Check sheet for the modelled part. Datum: model origin and axes. Units: mm. A direction names the side the tool comes from. Round coordinates to 2 decimals unless told otherwise and drop trailing zeros. Order: outer loops, then holes, each group sorted by start corner. A loop starts at its lowest first (then second) coordinate and runs counter-clockwise, first axis right, second up.
(1) Mould release check, pull along Y, two halves, no side actions. Record for faces 4 (the cylindrical face through (46.536, 9.274, 7.675)), 5 (the flat face through (34, 0, -1)), 6 (the cylindrical face through (24.5, 5.6, -5.6)): released by +Y, released by -Y, zero draft, split by the parting line, or undercut.
(2) Tool access check on faces 1 (the flat face through (10, 5.4, -8.5)), 2 (the flat face through (44, 2, 4)), 3 (the flat face through (31, 5, -11)). Record the directions out of +Z, -Z, +X, -X, +Y, -Y that give a thin tool (end or side, any length) a straight path to the whole face; none if there is none.
(3) Thickness scan on probe 1 along Y at (x, z) = (51, 5.75); probe 2 along X at (y, z) = (2.35, 8); probe 3 along Y at (x, z) = (40, -6). Record the ranges inside material, lowest first.
(4) Sectioned sample at B-B, the plane x = 22. Enter the section's corners in (y, z), and give its area (3 significant figures).
(5) Sectioned sample at D-D, the plane z = -4. Enter the section's corners in (x, y), and give its area (3 significant figures).
(6) Sectioned sample at A-A, the plane y = 7. Enter the section's corners in (x, z).
(7) Sectioned sample at C-C, the plane z = 8. Enter the section's corners in (x, y), and give its area (3 significant figures).
(8) Depth check by flat-ended pin: pin 1 (1 mm diameter, centred on y = 2, z = -8.5, fed in from +X); pin 2 (3.5 mm diameter, centred on x = 48, z = 8, fed in from -Y); pin 3 (1 mm diameter, centred on y = 1, z = 1.5, fed in from -X); pin 4 (1 mm diameter, centred on y = 4.5, z = 3.5, fed in from -X). Enter the tip coordinate at first touch or a pass-through.
```python
from build123d import *

# Parameters (mm, degrees)
BOSS_EXTRUDE1_DEPTH = 11
FILLET1_R           = 2
FILLET2_R           = 5
FILLET3_R           = 2
FILLET4_R           = 5
FILLET5_R           = 5.5
FILLET6_R           = 5.5
SKETCH2_W           = 22.197918088
SKETCH2_H           = 4
CUT_EXTRUDE1_DEPTH  = 11
SKETCH3_R           = 1.5
CUT_EXTRUDE2_DEPTH  = 11
SKETCH4_R           = 3
CUT_EXTRUDE3_DEPTH  = 31
SKETCH5_R           = 2.5
CUT_EXTRUDE4_DEPTH  = 31
SKETCH6_R           = 1.5
CUT_EXTRUDE5_DEPTH  = 31


with BuildPart() as part:
    # Sketch1 → Boss-Extrude1 (new body)
    with BuildSketch(Plane(origin=(0, 0, 0), x_dir=(1, 0, 0), z_dir=(0, 1, 0))):
        Polygon((0, 0), (0, 3), (10, 3), (10, 11), (55, 11), (55, -14), (44, -14), (44, 0), align=None)
    extrude(amount=BOSS_EXTRUDE1_DEPTH)

    # Fillet1
    fillet1_edges = [part.edges().sort_by_distance(p)[0] for p in [
        (0, 5.5, -3),
    ]]
    fillet(fillet1_edges, radius=FILLET1_R)

    # Fillet2
    fillet2_edges = [part.edges().sort_by_distance(p)[0] for p in [
        (10, 5.5, -3),
    ]]
    fillet(fillet2_edges, radius=FILLET2_R)

    # Fillet3
    fillet3_edges = [part.edges().sort_by_distance(p)[0] for p in [
        (10, 5.5, -11),
    ]]
    fillet(fillet3_edges, radius=FILLET3_R)

    # Fillet4
    fillet4_edges = [part.edges().sort_by_distance(p)[0] for p in [
        (55, 5.5, -11),
    ]]
    fillet(fillet4_edges, radius=FILLET4_R)

    # Fillet5
    fillet5_edges = [part.edges().sort_by_distance(p)[0] for p in [
        (44, 5.5, 14),
    ]]
    fillet(fillet5_edges, radius=FILLET5_R)

    # Fillet6
    fillet6_edges = [part.edges().sort_by_distance(p)[0] for p in [
        (55, 5.5, 14),
    ]]
    fillet(fillet6_edges, radius=FILLET6_R - 0.0001)  # a hair under: the kernel refuses the full size

    # Sketch2 → Cut-Extrude1 (cut)
    with BuildSketch(Plane.ZY.offset(-44)):
        with Locations((11.098959044, 5.5)):
            Rectangle(SKETCH2_W, SKETCH2_H)
    extrude(amount=-CUT_EXTRUDE1_DEPTH, mode=Mode.SUBTRACT)

    # Sketch3 → Cut-Extrude2 (cut)
    with BuildSketch(Plane(origin=(0, 11, 0), x_dir=(1, 0, 0), z_dir=(0, 1, 0))):
        with Locations(Location((48, -8, 0), (0, 0, 270))):
            Circle(SKETCH3_R)
    extrude(amount=-CUT_EXTRUDE2_DEPTH, mode=Mode.SUBTRACT)

    # Sketch4 → Cut-Extrude3 (cut)
    with BuildSketch(Plane(origin=(0, 0, -11), x_dir=(-1, 0, 0), z_dir=(0, 0, -1))):
        with Locations((-40, 5.5)):
            Circle(SKETCH4_R)
    extrude(amount=-CUT_EXTRUDE3_DEPTH, mode=Mode.SUBTRACT)

    # Sketch5 → Cut-Extrude4 (cut)
    with BuildSketch(Plane(origin=(0, 0, -11), x_dir=(-1, 0, 0), z_dir=(0, 0, -1))):
        with Locations((-22, 5.5)):
            Circle(SKETCH5_R)
    extrude(amount=-CUT_EXTRUDE4_DEPTH, mode=Mode.SUBTRACT)

    # Sketch6 → Cut-Extrude5 (cut)
    with BuildSketch(Plane(origin=(0, 11, 0), x_dir=(1, 0, 0), z_dir=(0, 1, 0))):
        with Locations(Location((50, 6, 0), (0, 0, 270))):
            Circle(SKETCH6_R)
    extrude(amount=-CUT_EXTRUDE5_DEPTH, mode=Mode.SUBTRACT)


solid = part.part
```
Derived:
1. face 4: zero draft
1. face 5: released by -Y
1. face 6: undercut
2. face 1: -Z, -X, +Y, -Y
2. face 2: +Z, -X, +Y, -Y
2. face 3: -Z, +X, -X, +Y, -Y
3. probe 1: y = 0 to 3.5, 7.5 to 11
3. probe 2: x = 44 to 46.5, 49.5 to 55
3. probe 3: y = 0 to 2.5, 8.5 to 11
4. outline: (0, -11) - (3, -11) - (3, 0) - (0, 0) - close; (8, -11) - (11, -11) - (11, 0) - (8, 0) - close
4. area: 66.0 mm2
5. outline: (8, 0) - (55, 0) - (55, 11) - (8, 11) - close; hole circle Ø5 at (22, 5.5); hole circle Ø6 at (40, 5.5)
5. area: 469 mm2
6. outline: (0, -1) arc R2 ccw to (2, -3) - (5, -3) arc R5 cw to (10, -8) - (10, -9) arc R2 ccw to (12, -11) - (20, -11) - (20, 0) - (0, 0) - close; (24, -11) - (37.4, -11) - (37.4, 0) - (24, 0) - close; (42.6, -11) - (50, -11) arc R5 ccw to (55, -6) - (55, 0) - (42.6, 0) - close; hole circle Ø3 at (50, -6)
7. outline: (44, 0) - (46.5, 0) - (46.5, 3.5) - (44, 3.5) - close; (44, 7.5) - (46.5, 7.5) - (46.5, 11) - (44, 11) - close; (49.5, 0) - (55, 0) - (55, 3.5) - (49.5, 3.5) - close; (49.5, 7.5) - (55, 7.5) - (55, 11) - (49.5, 11) - close
7. area: 56.0 mm2
8. pin 1: stops at x = 54.58
8. pin 2: stops at y = 0
8. pin 3: stops at x = 44
8. pin 4: passes through
